Source: CAD feature listing. Evaluate the final solid. Frame: model axes, mm. A direction names the side the tool comes from. Give positions to 0.01 mm unless a question says otherwise; leave off trailing zeros. Write each loop counter-clockwise with the first axis right and the second up, starting at its lowest first coordinate (ties: lowest second). Pieces come first, ordered by that corner, then holes. Notation, with made-up numbers: (24, 53.5) -> (81, 53.5) arc R10 cw to (81, 69.5) -> close; hole circle Ø2 at (-9.5, 36.25). An arc over 180 degrees is marked (long way). Use one line per item in the form item = value. Start each with the question number.
(1) Set-up query: faces 1 (the face through (36.41, 1.6, -6.58)), 2 (the face through (25.45, 3, -4)), 3 (the face through (19.5, 0.616, -14.946)), 4 (the face through (6.66, 4.26, -8.39)). Return all of +Z, -Z, +X, -X, +Y, -Y with unobstructed straight access to the full face (end or side cutting, diameter ignored); none if empty.
(2) Material intervals for line 1 along X through (y, z) = (0.7, -6.95); line 2 along X through (y, z) = (1.4, -7); line 3 along X through (y, z) = (2.1, -2), sorted ascending. Write a range as from..to.
(3) Cut plane A-A, the plane y = 4.1. Output: boundary loops of the cut face in (x, z), and give its area (3 significant figures).
(4) Cut plane C-C, the plane z = -11.25. Output: boundary loops of the cut face in (x, y).
(5) First-contact query: P1, Ø3, axis at x = 34.75, z = -6.95, coming from the -Y side (1 decimal); P2, Ø1, axis at x = 4.5, y = 4, coming from the -Z side. Flat tips, straight axial feed; report the tip coordinate or a pass-through.
(6) Cut plane B-B, the plane x = 34.75. Output: boundary loops of the cut face in (y, z), and give its area (3 significant figures).
(7) Draft query along X for faces 5 (the face through (6, 3, 0)), 6 (the face through (5.86, 1.6, -6.58)), 7 (the face through (0, 3, -4)). Return one class per face: pulls with the +X half, pulls with the -X half, needs draft (parallel to the pull), parting line crosses it, or undercut.
(8) Cut plane D-D, the plane x = 12. Output: boundary loops of the cut face in (y, z).
from build123d import *

# Parameters (mm, degrees)
ESBO_O1_R                = 1.7
RESSALTO_EXTRUS_O1_DEPTH = 5.25
ESBO_O2_R                = 7.95
CORTE_EXTRUS_O1_DEPTH    = 1.25
FILETE1_R                = 4
FILETE2_R                = 8
CORTE_EXTRUS_O2_DEPTH    = 2


with BuildPart() as part:
    # Esboço1 → Ressalto-extrusão1 (new body)
    with BuildSketch(Plane(origin=(0, 0, 0), x_dir=(1, 0, 0), z_dir=(0, 1, 0))):
        with BuildLine():
            Line((13.05, 0), (13.05, 7))
            ThreePointArc((13.05, 7), (19.25, 13.2), (25.45, 7))
            Line((25.45, 7), (25.45, 0))
            Line((25.45, 0), (44, 0))
            Line((44, 0), (44, 19))
            Line((44, 19), (17.2, 19))
            Line((17.2, 19), (0, 9.5))
            Line((0, 9.5), (0, 0))
            Line((0, 0), (13.05, 0))
        make_face()
        with Locations(Location((4.2, 6.95, 0), (0, 0, 90))):
            Circle(ESBO_O1_R, mode=Mode.SUBTRACT)
        with Locations(Location((34.75, 6.95, 0), (0, 0, 90))):
            Circle(ESBO_O1_R, mode=Mode.SUBTRACT)
        with Locations(Location((40.05, 14.337730871, 0), (0, 0, 90))):
            Circle(ESBO_O1_R, mode=Mode.SUBTRACT)
    extrude(amount=RESSALTO_EXTRUS_O1_DEPTH)

    # Esboço2 → Corte-extrusão1 (cut)
    with BuildSketch(Plane(origin=(0, 0, 0), x_dir=(1, 0, 0), z_dir=(0, 1, 0))):
        with Locations((19.25, 7)):
            Circle(ESBO_O2_R)
    extrude(amount=CORTE_EXTRUS_O1_DEPTH, mode=Mode.SUBTRACT)

    # Filete1
    filete1_edges = [part.edges().sort_by_distance(p)[0] for p in [
        (0, 2.625, -9.5),
    ]]
    fillet(filete1_edges, radius=FILETE1_R)

    # Filete2
    filete2_edges = [part.edges().sort_by_distance(p)[0] for p in [
        (17.2, 2.625, -19),
    ]]
    fillet(filete2_edges, radius=FILETE2_R)

    # Esboço3 → Corte-extrusão2 (cut)
    with BuildSketch(Plane(origin=(0, 5.25, 0), x_dir=(-1, 0, 0), z_dir=(0, -1, 0))):
        Polygon((-31.459103466, 6.95), (-33.104551733, 9.8), (-36.395448267, 9.8), (-38.040896534, 6.95), (-36.395448267, 4.1), (-33.104551733, 4.1), align=None)
        Polygon((-0.909103466, 6.95), (-2.554551733, 9.8), (-5.845448267, 9.8), (-7.490896534, 6.95), (-5.845448267, 4.1), (-2.554551733, 4.1), align=None)
    extrude(amount=CORTE_EXTRUS_O2_DEPTH, mode=Mode.SUBTRACT)


solid = part.part
Geometry says:
q1.face_1 = +Y, -Y
q1.face_2 = +Z, +Y, -Y
q1.face_3 = -Y
q1.face_4 = +Y
q2.line_1 = 0..2.5, 5.9..11.3, 27.2..33.05, 36.45..44
q2.line_2 = 0..2.5, 5.9..13.05, 25.45..33.05, 36.45..44
q2.line_3 = 0..13.05, 25.45..44
q3.outline = (0, -7.14) arc R4 ccw to (2.07, -10.64) -> (15.39, -18) arc R8 ccw to (19.26, -19) -> (44, -19) -> (44, 0) -> (25.45, 0) -> (25.45, -7) arc R6.2 cw to (13.05, -7) -> (13.05, 0) -> (0, 0) -> close; hole (0.91, -6.95) -> (2.55, -9.8) -> (5.85, -9.8) -> (7.49, -6.95) -> (5.85, -4.1) -> (2.55, -4.1) -> close; hole (31.46, -6.95) -> (33.1, -9.8) -> (36.4, -9.8) -> (38.04, -6.95) -> (36.4, -4.1) -> (33.1, -4.1) -> close; hole circle Ø3.4 at (40.05, -14.34)
q3.area = 541 mm^2
q4.outline = (3.17, 0) -> (12.53, 0) -> (12.53, 1.25) -> (14.74, 1.25) -> (14.74, 5.25) -> (3.17, 5.25) -> close; (23.76, 1.25) -> (25.97, 1.25) -> (25.97, 0) -> (44, 0) -> (44, 5.25) -> (23.76, 5.25) -> close
q5.P1 = through
q5.P2 = -12.26
q6.outline = (0, -19) -> (5.25, -19) -> (5.25, -9.8) -> (3.25, -9.8) -> (3.25, -8.65) -> (0, -8.65) -> close; (0, -5.25) -> (3.25, -5.25) -> (3.25, -4.1) -> (5.25, -4.1) -> (5.25, 0) -> (0, 0) -> close
q6.area = 77.3 mm^2
q7.face_5 = needs draft
q7.face_6 = undercut
q7.face_7 = pulls with the -X half
q8.outline = (0, -16.13) -> (5.25, -16.13) -> (5.25, 0) -> (0, 0) -> (0, -3.74) -> (1.25, -3.74) -> (1.25, -10.26) -> (0, -10.26) -> close
